```python
from build123d import *

# Parameters (mm, degrees)
F0_R     = 1.5
F0_R_2   = 19.5
F1_DEPTH = 5
F2_R     = 1.5
F3_DEPTH = 5


with BuildPart() as f1:
    # F0 (on Right) → F1 (new body)
    with BuildSketch(Plane.YZ):
        Polygon((0, 49), (0, 0), (73.25, 0), (73.25, 5), (85.25, 5), (85.25, 0), (158.5, 0), (158.5, 49), align=None)
        with Locations((8, 2.5)):
            Circle(F0_R, mode=Mode.SUBTRACT)
        with Locations((55.5, 2.5)):
            Circle(F0_R, mode=Mode.SUBTRACT)
        with Locations((2.5, 24.5)):
            Circle(F0_R, mode=Mode.SUBTRACT)
        with Locations((29.5, 22)):
            Circle(F0_R_2, mode=Mode.SUBTRACT)
        with Locations((103, 2.5)):
            Circle(F0_R, mode=Mode.SUBTRACT)
        with Locations((150.5, 2.5)):
            Circle(F0_R, mode=Mode.SUBTRACT)
        with Locations((156, 24.5)):
            Circle(F0_R, mode=Mode.SUBTRACT)
    extrude(amount=F1_DEPTH)

    # F2 (on face) → F3 (cut)
    with BuildSketch(Plane.XY.offset(49)):
        with Locations((2.5, 55.5)):
            Circle(F2_R)
        with Locations((2.5, 103)):
            Circle(F2_R)
    extrude(amount=-F3_DEPTH, mode=Mode.SUBTRACT)


solid = f1.part
```
The listing builds one solid part. Answer for the finished solid, in the listing's coordinates (mm). A direction names the side the tool comes from. Round coordinates to 2 decimals unless told otherwise and drop trailing zeros. Write each loop counter-clockwise with the first axis right and the second up, starting at its lowest first coordinate (ties: lowest second). Pieces come first, ordered by that corner, then holes. Notation, with made-up numbers: (41, 50.25) -> (47, 50.25) arc R38 ccw to (47, 89.25) -> close; hole circle Ø9 at (21, 32). An arc over 180 degrees is marked (long way). Answer as a JSON object with one key per item and string values. Group by question number.
Q1. Section D-D (x = 3.1) is taken. Write down the section's boundary in (y, z), plus the area to 3 significant figures.
Q2. Section A-A (y = 29.5) is taken. Write down the section's boundary in (x, z).
Q3. Determine the mould class of faces 4 (the face through (5, 96, 25)), 5 (the face through (2, 56, 44)), 6 (the face through (2.5, 47.5, 14.5)) for opening direction X: pulls with the +X half, pulls with the -X half, needs draft (parallel to the pull), parting line crosses it, or undercut.
Q4. Section B-B (z = 17) is taken. Write down the section's boundary in (x, y), plus the area to 3 significant figures.
Q5. Section C-C (z = 24.5) is taken. Write down the section's boundary in (x, y).
Q6. Straight lines are drawn through the part: line 1 along Y through (x, z) = (2.5, 47.15); line 2 along Z through (x, y) = (3, 103); line 3 along X through (y, z) = (103, 46.2). For each, find the intervals that lie inside material, in ascending order.
Q7. Each of these flat-tipped pins is pushed along its axis until it touches: pin 1 Ø1.5 at (x, y) = (3, 82) entering from -Z; pin 2 Ø0.9 at (x, y) = (2, 102.5) entering from +Z. Where does it stop, or does it pass through?
Q8. Which of the six approach directions +Z, -Z, +X, -X, +Y, -Y give full straight-line access (tool end or side, diameter ignored) to faces 1 (the face through (2.5, 6.8, 1.6)), 2 (the face through (2, 103, 44)), 3 (the face through (2, 85.25, 3))?
Check values:
{
 "1": {"outline": "(0, 0) -> (73.25, 0) -> (73.25, 5) -> (85.25, 5) -> (85.25, 0) -> (158.5, 0) -> (158.5, 49) -> (104.37, 49) -> (104.37, 44) -> (101.63, 44) -> (101.63, 49) -> (56.87, 49) -> (56.87, 44) -> (54.13, 44) -> (54.13, 49) -> (0, 49) -> close; hole circle Ø3 at (2.5, 24.5); hole circle Ø3 at (8, 2.5); hole circle Ø39 at (29.5, 22); hole circle Ø3 at (55.5, 2.5); hole circle Ø3 at (103, 2.5); hole circle Ø3 at (150.5, 2.5); hole circle Ø3 at (156, 24.5)", "area": "6,440 mm^2"},
 "2": {"outline": "(0, 0) -> (5, 0) -> (5, 2.5) -> (0, 2.5) -> close; (0, 41.5) -> (5, 41.5) -> (5, 49) -> (0, 49) -> close"},
 "3": {"face 4": "pulls with the +X half", "face 5": "undercut", "face 6": "needs draft"},
 "4": {"outline": "(0, 0) -> (5, 0) -> (5, 10.65) -> (0, 10.65) -> close; (0, 48.35) -> (5, 48.35) -> (5, 158.5) -> (0, 158.5) -> close", "area": "604 mm^2"},
 "5": {"outline": "(0, 0) -> (5, 0) -> (5, 1) -> (0, 1) -> close; (0, 4) -> (5, 4) -> (5, 10.16) -> (0, 10.16) -> close; (0, 48.84) -> (5, 48.84) -> (5, 154.5) -> (0, 154.5) -> close; (0, 157.5) -> (5, 157.5) -> (5, 158.5) -> (0, 158.5) -> close"},
 "6": {"line 1": "0 to 54, 57 to 101.5, 104.5 to 158.5", "line 2": "0 to 1, 4 to 44", "line 3": "0 to 1, 4 to 5"},
 "7": {"pin 1": "z = 5", "pin 2": "z = 44"},
 "8": {"face 1": "+X, -X", "face 2": "+Z", "face 3": "-Z, +X, -X"}
}
